Verification items for the finished model (mm, model axes). A direction names the side the tool comes from. Round coordinates to 2 decimals unless told otherwise and drop trailing zeros. Loops run counter-clockwise (first coordinate to the right, second up) from the corner with the lowest first, then second, coordinate; pieces in that order, holes last. Notation, with made-up numbers: (-30, 44) - (-17, 44) arc R19 cw to (-17, 64) - close; hole circle Ø3 at (33, 5.25). An arc over 180 degrees is marked (long way). Use a Markdown table: item, result. Add a question column.
```python
from build123d import *

# Parameters (mm, degrees)
F0_W     = 914.4
F0_H     = 304.8
F1_DEPTH = 12.7
F2_W     = 914.4
F2_H     = 11.938
F3_DEPTH = 101.6
F4_R     = 3.3734375
F5_DEPTH = 25.4
F6_R     = 3.3734375
F7_DEPTH = 327.66
F8_R     = 1.984375
F9_DEPTH = 9.525


with BuildPart() as f1:
    # F0 (on Top) → F1 (new body)
    with BuildSketch(Plane.XY):
        with Locations((457.2, 152.4)):
            Rectangle(F0_W, F0_H)
    extrude(amount=F1_DEPTH)

    # F2 (on face) → F3 (join)
    with BuildSketch(Plane.XY.offset(12.7)):
        with Locations((457.2, 5.969)):
            Rectangle(F2_W, F2_H)
        with Locations((457.2, 298.831)):
            Rectangle(F2_W, F2_H)
    extrude(amount=F3_DEPTH)

    # F4 (on face) → F5 (cut)
    with BuildSketch(Plane.XY.offset(12.7)):
        with Locations((25.4, 241.3)):
            Circle(F4_R)
        with Locations((279.4, 241.3)):
            Circle(F4_R)
        with Locations((279.4, 63.5)):
            Circle(F4_R)
        with Locations((635, 241.3)):
            Circle(F4_R)
        with Locations((889, 241.3)):
            Circle(F4_R)
        with Locations((635, 63.5)):
            Circle(F4_R)
        with Locations((889, 63.5)):
            Circle(F4_R)
        with Locations((25.4, 63.5)):
            Circle(F4_R)
    extrude(amount=-F5_DEPTH, mode=Mode.SUBTRACT)

    # F6 (on face) → F7 (cut, symmetric)
    with BuildSketch(Plane(origin=(0, 11.938, 0), x_dir=(-1, 0, 0), z_dir=(0, 1, 0))):
        with Locations((-889, 25.4)):
            Circle(F6_R)
        with Locations((-635, 25.4)):
            Circle(F6_R)
        with Locations((-279.4, 25.4)):
            Circle(F6_R)
        with Locations((-25.4, 25.4)):
            Circle(F6_R)
    extrude(amount=F7_DEPTH, both=True, mode=Mode.SUBTRACT)

    # F8 (on face) → F9 (cut)
    with BuildSketch(Plane(origin=(0, 0, 0), x_dir=(1, 0, 0), z_dir=(0, 0, -1))):
        with Locations((25.4, -279.4)):
            Circle(F8_R)
        with Locations((889, -279.4)):
            Circle(F8_R)
        with Locations((457.2, -279.4)):
            Circle(F8_R)
        with Locations((889, -25.4)):
            Circle(F8_R)
        with Locations((457.2, -25.4)):
            Circle(F8_R)
        with Locations((25.4, -25.4)):
            Circle(F8_R)
    extrude(amount=-F9_DEPTH, mode=Mode.SUBTRACT)


solid = f1.part
```
Q1. Release check for a two-part mould opening along Y. For faces 3 (the face through (451, 154, 12.7)), 4 (the face through (451, 0, 56)), 5 (the face through (0, 152, 10)) record: +Y half, -Y half, draft (parallel to the pull), parting line (faces both ways), or undercut.
Q2. Set-up check for faces 1 (the face through (451, 292.862, 63)), 2 (the face through (451, 304.8, 56)): record each of +Z, -Z, +X, -X, +Y, -Y from which the full face is reachable in a straight line by a thin tool's end or side.
Q3. Section check C-C on y = 168. Record the cut outline in (x, z).
Q4. Thickness scan on line 1 along X through (y, z) = (241.3, 9); line 2 along X through (y, z) = (300, 25); line 3 along Y through (x, z) = (635, 5.75). Record the ranges inside material, lowest first.
Q5. Section check B-B on x = 413. Record the cut outline in (y, z).
Q6. Go/stop test with flat-tipped pins: pin 1 Ø3 at (x, y) = (889, 279.4) entering from +Z; pin 2 Ø9 at (x, z) = (25.4, 25.4) entering from +Y; pin 3 Ø2.5 at (x, y) = (457.2, 25.4) entering from -Z (3 decimals). Record where each tip stops, or that it passes through.
Q7. Section check A-A on z = 102. Record the cut outline in (x, y), plus the area to 3 significant figures.
Determined:
| question | item | result |
|---|---|---|
| 1 | face 3 | undercut |
| 1 | face 4 | -Y half |
| 1 | face 5 | draft |
| 2 | face 1 | +Z, +X, -X |
| 2 | face 2 | +Z, -Z, +X, -X, +Y |
| 3 | outline | (0, 0) - (914.4, 0) - (914.4, 12.7) - (0, 12.7) - close |
| 4 | line 1 | x = 0 to 22.03, 28.77 to 276.03, 282.77 to 631.63, 638.37 to 885.63, 892.37 to 914.4 |
| 4 | line 2 | x = 0 to 22.05, 28.75 to 276.05, 282.75 to 631.65, 638.35 to 885.65, 892.35 to 914.4 |
| 4 | line 3 | y = 0 to 60.13, 66.87 to 237.93, 244.67 to 304.8 |
| 5 | outline | (0, 0) - (304.8, 0) - (304.8, 114.3) - (292.86, 114.3) - (292.86, 12.7) - (11.94, 12.7) - (11.94, 114.3) - (0, 114.3) - close |
| 6 | pin 1 | stops at z = 12.7 |
| 6 | pin 2 | stops at y = 304.8 |
| 6 | pin 3 | stops at z = 9.525 |
| 7 | outline | (0, 0) - (914.4, 0) - (914.4, 11.94) - (0, 11.94) - close; (0, 292.86) - (914.4, 292.86) - (914.4, 304.8) - (0, 304.8) - close |
| 7 | area | 21,800 mm² |
